from build123d import *

# Parameters (mm, degrees)
F0_W     = 95
F0_H     = 26
F1_DEPTH = 7.5
F3_D     = 6.4
F4_SIZE  = 3


with BuildPart() as f1:
    # F0 (on Top) → F1 (new body, symmetric)
    with BuildSketch(Plane.XY):
        Rectangle(F0_W, F0_H)
    extrude(amount=F1_DEPTH, both=True)

    # F3 (through all)
    with Locations(Plane.XY.offset(7.5)):
        with Locations((-40, 7), (-40, -7), (40, 7), (40, -7)):
            Hole(F3_D / 2)

    # F4
    f4_edges = [f1.edges().sort_by_distance(p)[0] for p in [
        (-47.5, 13, 0),
        (47.5, 13, 0),
        (47.5, -13, 0),
        (-47.5, -13, 0),
    ]]
    chamfer(f4_edges, length=F4_SIZE)


solid = f1.part
Build history of the part. All positions in model axes, mm. Give positions to 0.01 mm unless a question says otherwise; leave off trailing zeros. Order: outer loops, then holes, each group sorted by start corner. A loop starts at its lowest first (then second) coordinate and runs counter-clockwise, first axis right, second up. Notation, with made-up numbers: M 75,3.25 L 104,3.25 A28 ccw 104,23.25 Z; hole C -13.5,74.5 d7. An arc over 180 degrees is marked long. Put each result on its own line as item: value.
Item 1: Wall check: probe 1 along Y at (x, z) = (-40, -2.75); probe 2 along X at (y, z) = (-9.75, -5.5); probe 3 along X at (y, z) = (4.5, 6). Give the ranges that are in metal, low to high.
Results are:
probe 1: -13 to -10.2, -3.8 to 3.8, 10.2 to 13
probe 2: -47.5 to -41.64, -38.36 to 38.36, 41.64 to 47.5
probe 3: -47.5 to -42, -38 to 38, 42 to 47.5
Item 2: Cut at A-A on y = 7. Write the cut outline in (x, z), then the cut area to 3 significant figures.
Results are:
outline: M -47.5,-7.5 L -43.2,-7.5 L -43.2,7.5 L -47.5,7.5 Z; M -36.8,-7.5 L 36.8,-7.5 L 36.8,7.5 L -36.8,7.5 Z; M 43.2,-7.5 L 47.5,-7.5 L 47.5,7.5 L 43.2,7.5 Z
area: 1,230 mm2
Item 3: Cut at B-B on z = -6. Write the cut outline in (x, y), then the cut area to 3 significant figures.
Results are:
outline: M -47.5,-10 L -44.5,-13 L 44.5,-13 L 47.5,-10 L 47.5,10 L 44.5,13 L -44.5,13 L -47.5,10 Z; hole C -40,-7 d6.4; hole C -40,7 d6.4; hole C 40,-7 d6.4; hole C 40,7 d6.4
area: 2,320 mm2
Item 4: Cut at C-C on x = -40. Write the cut outline in (y, z).
Results are:
outline: M -13,-7.5 L -10.2,-7.5 L -10.2,7.5 L -13,7.5 Z; M -3.8,-7.5 L 3.8,-7.5 L 3.8,7.5 L -3.8,7.5 Z; M 10.2,-7.5 L 13,-7.5 L 13,7.5 L 10.2,7.5 Z
Item 5: Pull direction Y, two halves, no side cores. Call faces 1 (the face through (-46, 11.5, 0.1)), 2 (the face through (42.36, 9.16, -0.11)), 3 (the face through (-1, 0, -7.5)): +Y half, -Y half, draft (parallel to the pull), parting line (faces both ways), or undercut.
Results are:
face 1: +Y half
face 2: undercut
face 3: draft
